```python
from build123d import *

# Parameters (mm, degrees)
BOSS_EXTRUDE1_START = 12
SKETCH1_R           = 4
BOSS_EXTRUDE1_DEPTH = 17
BOSS_EXTRUDE2_START = 12
SKETCH2_R           = 4.6
BOSS_EXTRUDE2_DEPTH = 72
BOSS_EXTRUDE3_START = 49
SKETCH3_R           = 6
BOSS_EXTRUDE3_DEPTH = 4


with BuildPart() as part:
    # Sketch1 → Boss-Extrude1 (new body)
    with BuildSketch(Plane.XY.offset(BOSS_EXTRUDE1_START)):
        Circle(SKETCH1_R)
    extrude(amount=-BOSS_EXTRUDE1_DEPTH)

    # Sketch2 → Boss-Extrude2 (add)
    with BuildSketch(Plane.XY.offset(BOSS_EXTRUDE2_START)):
        Circle(SKETCH2_R)
    extrude(amount=BOSS_EXTRUDE2_DEPTH)

    # Sketch3 → Boss-Extrude3 (add)
    with BuildSketch(Plane.XY.offset(BOSS_EXTRUDE3_START)):
        Circle(SKETCH3_R)
    extrude(amount=-BOSS_EXTRUDE3_DEPTH)


solid = part.part
```
CAD build for the part. Positions are in the model's coordinates, mm. A direction names the side the tool comes from. Round coordinates to 2 decimals unless told otherwise and drop trailing zeros. Order: outer loops, then holes, each group sorted by start corner. A loop starts at its lowest first (then second) coordinate and runs counter-clockwise, first axis right, second up. Notation, with made-up numbers: (13.25, 54.25) - (29.25, 54.25) arc R17 cw to (29.25, 75.25) - close; hole circle Ø4 at (19, 31). An arc over 180 degrees is marked (long way). Answer in a Markdown table with one row per item. Add a question column.
(1) Band-saw the part on D-D on z = 18.5. List the corners of the cut face in (x, y).
(2) Band-saw the part on C-C on z = 7.5. List the corners of the cut face in (x, y), and give its area (3 significant figures).
(3) Band-saw the part on B-B on y = 3. List the corners of the cut face in (x, z), and give its area (3 significant figures).
(4) Band-saw the part on A-A on x = 0. List the corners of the cut face in (y, z).
(5) Probe L1, parallel to Z at x = 5.25, y = -1.75; L2, parallel to Y at x = -1.75, z = 34.5; L3, parallel to X at y = 0, z = 80. List the from-to ranges inside material, lowest first. Write a range as [from, to].
(6) Drop flat-ended pins along their axis: pin 1 Ø1 at (x, z) = (-2.5, 4) entering from -Y; pin 2 Ø1.5 at (x, z) = (0.5, 55) entering from -Y; pin 3 Ø5 at (x, z) = (0.5, 27.5) entering from +Y. Give the stop position or say it passes through.
(7) 3-axis set-ups, long thin cutter, end or side, ignore diameter. For faces 1 (the face through (-3.65, -2.8, 28.27)), 2 (the face through (3, -4, 49)), 3 (the face through (0, 0, -5)): which of +Z, -Z, +X, -X, +Y, -Y reach the whole face in a straight line?
Data:
| question | item | result |
|---|---|---|
| 1 | outline | circle Ø9.2 at (0, 0) |
| 2 | outline | circle Ø8 at (0, 0) |
| 2 | area | 50.3 mm^2 |
| 3 | outline | (-5.2, 45) - (-3.49, 45) - (-3.49, 12) - (-2.65, 12) - (-2.65, -5) - (2.65, -5) - (2.65, 12) - (3.49, 12) - (3.49, 45) - (5.2, 45) - (5.2, 49) - (3.49, 49) - (3.49, 84) - (-3.49, 84) - (-3.49, 49) - (-5.2, 49) - close |
| 3 | area | 606 mm^2 |
| 4 | outline | (-6, 45) - (-4.6, 45) - (-4.6, 12) - (-4, 12) - (-4, -5) - (4, -5) - (4, 12) - (4.6, 12) - (4.6, 45) - (6, 45) - (6, 49) - (4.6, 49) - (4.6, 84) - (-4.6, 84) - (-4.6, 49) - (-6, 49) - close |
| 5 | L1 | z = [45, 49] |
| 5 | L2 | y = [-4.25, 4.25] |
| 5 | L3 | x = [-4.6, 4.6] |
| 6 | pin 1 | stops at y = -3.46 |
| 6 | pin 2 | stops at y = -4.6 |
| 6 | pin 3 | stops at y = 4.6 |
| 7 | face 1 | -Z |
| 7 | face 2 | +Z |
| 7 | face 3 | -Z, +X, -X, +Y, -Y |
